Read the model definition and answer for the solid it produces. Units are mm, in the model's axes. A direction names the side the tool comes from. Coordinates: 2 decimals unless noted, no trailing zeros. Write each loop counter-clockwise with the first axis right and the second up, starting at its lowest first coordinate (ties: lowest second). Pieces come first, ordered by that corner, then holes.
1) The part is cut by section D-D (y = 4). Determine the outline of the cut face in (x, z) (3 decimals), then the cut area to 3 significant figures.
2) The part is cut by section A-A (y = 6.75). Determine the outline of the cut face in (x, z) (3 decimals).
3) The part is cut by section B-B (z = -3.5). Determine the outline of the cut face in (x, y) (3 decimals), then the cut area to 3 significant figures.
4) Determine the mould class of faces 1 (the face through (-4.225, 7, 0)), 2 (the face through (0, 10, 0)), 3 (the face through (2.599, 6.014, 4.234)), 4 (the face through (0, 0, 0)) for opening direction Y: +Y half, -Y half, draft (parallel to the pull), parting line (faces both ways), or undercut.
5) The part is cut by section C-C (x = -6.75). Determine the outline of the cut face in (y, z).
6) Find the intervals of material crossed by line 1 (Y direction, x = 0.5, z = 0); line 2 (X direction, y = 6.75, z = -1.75) (3 decimals); line 3 (Z direction, x = 1.75, y = 5), in increasing order.
7) Each of these flat-tipped pins is pushed along its axis until it touches: pin 1 Ø1.8 at (y, z) = (5, 0) entering from -X; pin 2 Ø5 at (y, z) = (5, 0) entering from -X (3 decimals). Where does it stop, or does it pass through?
8) Which of the six approach directions +Z, -Z, +X, -X, +Y, -Y give full straight-line access (tool end or side, diameter ignored) to faces 5 (the face through (6.42, 5.07, -1.5)), 6 (the face through (-5.14, 3.84, -2.05))?
from build123d import *

# Parameters (mm, degrees)
SKETCH1_W           = 16.41
SKETCH1_H           = 13.7
BOSS_EXTRUDE1_DEPTH = 10
SKETCH2_R           = 1.5
CUT_EXTRUDE1_DEPTH  = 19.841762789
SKETCH3_R           = 1.5
CUT_EXTRUDE2_DEPTH  = 21.401240158
SKETCH5_W           = 0.18
SKETCH5_H           = 13.7
CUT_EXTRUDE4_DEPTH  = 15.637094145
CUT_EXTRUDE3_DEPTH  = 1.8
SKETCH6_W           = 1.8
SKETCH6_H           = 5.438639536
CUT_EXTRUDE5_DEPTH  = 5


with BuildPart() as part:
    # Sketch1 → Boss-Extrude1 (new body)
    with BuildSketch(Plane(origin=(0, 0, 0), x_dir=(1, 0, 0), z_dir=(0, 1, 0))):
        Rectangle(SKETCH1_W, SKETCH1_H)
    extrude(amount=BOSS_EXTRUDE1_DEPTH)

    # Sketch2 → Cut-Extrude1 (cut, through all)
    with BuildSketch(Plane.XY.offset(6.85)):
        with Locations((3.705, 5)):
            Circle(SKETCH2_R)
    extrude(amount=-CUT_EXTRUDE1_DEPTH, mode=Mode.SUBTRACT)

    # Sketch3 → Cut-Extrude2 (cut, through all)
    with BuildSketch(Plane.ZY.offset(8.205)):
        with Locations((0, 5)):
            Circle(SKETCH3_R)
    extrude(amount=-CUT_EXTRUDE2_DEPTH, mode=Mode.SUBTRACT)

    # Sketch5 → Cut-Extrude4 (cut, through all)
    with BuildSketch(Plane(origin=(0, 10, 0), x_dir=(1, 0, 0), z_dir=(0, 1, 0))):
        with Locations((-8.115, 0)):
            Rectangle(SKETCH5_W, SKETCH5_H)
    extrude(amount=-CUT_EXTRUDE4_DEPTH, mode=Mode.SUBTRACT)

    # Sketch4 → Cut-Extrude3 (cut)
    with BuildSketch(Plane.ZY.offset(6.025)):
        Polygon((2.719319768, 5), (1.359659884, 7.355), (-1.359659884, 7.355), (-2.719319768, 5), (-1.359659884, 2.645), (1.359659884, 2.645), align=None)
    extrude(amount=-CUT_EXTRUDE3_DEPTH, mode=Mode.SUBTRACT)

    # Sketch6 → Cut-Extrude5 (cut)
    with BuildSketch(Plane(origin=(0, 10, 0), x_dir=(1, 0, 0), z_dir=(0, 1, 0))):
        with Locations((-5.125, 0)):
            Rectangle(SKETCH6_W, SKETCH6_H)
    extrude(amount=-CUT_EXTRUDE5_DEPTH, mode=Mode.SUBTRACT)


solid = part.part
Reported:
1. outline: (-8.025, -6.85) - (2.587, -6.85) - (2.587, -1.118) - (-4.225, -1.118) - (-4.225, -2.142) - (-6.025, -2.142) - (-6.025, -1.118) - (-8.025, -1.118) - close; (-8.025, 1.118) - (-6.025, 1.118) - (-6.025, 2.142) - (-4.225, 2.142) - (-4.225, 1.118) - (2.587, 1.118) - (2.587, 6.85) - (-8.025, 6.85) - close; (4.823, -6.85) - (8.205, -6.85) - (8.205, -1.118) - (4.823, -1.118) - close; (4.823, 1.118) - (8.205, 1.118) - (8.205, 6.85) - (4.823, 6.85) - close
1. area: 157 mm2
2. outline: (-8.025, -6.85) - (8.205, -6.85) - (8.205, 6.85) - (-8.025, 6.85) - close; hole (-6.025, -2.719) - (-4.225, -2.719) - (-4.225, 2.719) - (-6.025, 2.719) - close
3. outline: (-8.025, 0) - (8.205, 0) - (8.205, 10) - (-8.025, 10) - close; hole circle Ø3 at (3.705, 5)
3. area: 155 mm2
4. face 1: draft
4. face 2: +Y half
4. face 3: undercut
4. face 4: -Y half
5. outline: (0, -6.85) - (10, -6.85) - (10, 6.85) - (0, 6.85) - close; hole circle Ø3 at (5, 0)
6. line 1: y = 0 to 3.5, 6.5 to 10
6. line 2: x = -8.025 to -6.025, -4.225 to 8.205
6. line 3: z = -6.85 to -1.5, 1.5 to 6.85
7. pin 1: passes through
7. pin 2: stops at x = -8.025
8. face 5: +X, -X
8. face 6: +Y
